Can you work these out from the model? Positions are in its coordinate system, mm. Face numbers are marked on the shaded views. Round coordinates to 2 decimals unless told otherwise and drop trailing zeros. Order: outer loops, then holes, each group sorted by start corner. A loop starts at its lowest first (then second) coordinate and runs counter-clockwise, first axis right, second up. Notation, with made-up numbers: (28.5, 6.25) -> (42.5, 6.25) arc R36 ccw to (42.5, 42.25) -> close; hole circle Ø2 at (11.25, 25.25). An arc over 180 degrees is marked (long way). Use a Markdown table: item, result. Add a question column.
Q1. I'm going to push flat-ended pins straight in: pin 1 Ø8 at (y, z) = (6, -11.5) entering from +X; pin 2 Ø12 at (y, z) = (6, -18) entering from +X; pin 3 Ø3 at (x, y) = (-14, 5.5) entering from -Z. Where does each tip first touch, or does it pass through?
Q2. I need wall thicknesses on line 1 along Z through (x, y) = (0, 15.75); line 2 along X through (y, z) = (9.5, -4); line 3 along Z through (x, y) = (8.5, 17.75). Which ranges of each line are inside material? Lowest first, please. Write a range as [from, to].
Q3. If we section it at C-C on y = 17.5: List the corners of the cut face in (x, z) for me, plus the area to 3 significant figures.
Q4. We'd pull the mould along X, two halves only. Please class the marked faces 1, 2, 3 and 4: +X half, -X half, draft (parallel to the pull), parting line (faces both ways), or undercut.
Q5. If we section it at D-D on x = 38: List the corners of the cut face in (y, z) for me, plus the area to 3 significant figures.
Q6. If we section it at A-A on z = 0: List the corners of the cut face in (x, y) for me, plus the area to 3 significant figures.
Q7. If we section it at B-B on x = 0: List the corners of the cut face in (y, z) for me, plus the area to 3 significant figures.
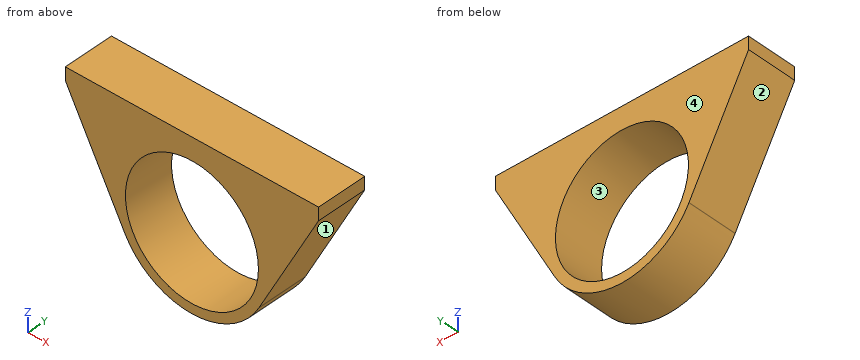
```python
from build123d import *

# Parameters (mm, degrees)
SKETCH1_R           = 30
BOSS_EXTRUDE1_DEPTH = 20
SKETCH2_R           = 26.25
CUT_EXTRUDE1_DEPTH  = 20


with BuildPart() as part:
    # Sketch1 → Boss-Extrude1 (new body)
    with BuildSketch(Plane(origin=(0, 0, 0), x_dir=(1, 0, 0), z_dir=(0, 1, 0))):
        Circle(SKETCH1_R)
        with BuildLine():
            Line((-26.470588235, 14.117647059), (-50, -30))
            Line((-50, -30), (-50, -35))
            Line((-50, -35), (50, -35))
            Line((50, -35), (50, -30))
            Line((50, -30), (26.470588235, 14.117647059))
            ThreePointArc((26.470588235, 14.117647059), (29.104275004, 7.276068751), (30, 0))
            ThreePointArc((30, 0), (-7.276068751, -29.104275004), (-26.470588235, 14.117647059))
        make_face()
    extrude(amount=BOSS_EXTRUDE1_DEPTH)

    # Sketch2 → Cut-Extrude1 (cut)
    with BuildSketch(Plane(origin=(0, 0, 0), x_dir=(1, 0, 0), z_dir=(0, 1, 0))):
        Circle(SKETCH2_R)
    extrude(amount=CUT_EXTRUDE1_DEPTH, mode=Mode.SUBTRACT)


solid = part.part
```
Answer below:
| question | item | result |
|---|---|---|
| 1 | pin 1 | x = 30 |
| 1 | pin 2 | x = 27.6 |
| 1 | pin 3 | z = -27.27 |
| 2 | line 1 | [-30, -26.25], [26.25, 35] |
| 2 | line 2 | [-31.87, -25.94], [25.94, 31.87] |
| 2 | line 3 | [-28.77, -24.84], [24.84, 35] |
| 3 | outline | (-50, 30) -> (-26.47, -14.12) arc R30 ccw to (26.47, -14.12) -> (50, 30) -> (50, 35) -> (-50, 35) -> close; hole circle Ø52.5 at (0, 0) |
| 3 | area | 2,310 mm² |
| 4 | face 1 | +X half |
| 4 | face 2 | -X half |
| 4 | face 3 | undercut |
| 4 | face 4 | draft |
| 5 | outline | (0, 7.5) -> (20, 7.5) -> (20, 35) -> (0, 35) -> close |
| 5 | area | 550 mm² |
| 6 | outline | (-34, 0) -> (-26.25, 0) -> (-26.25, 20) -> (-34, 20) -> close; (26.25, 0) -> (34, 0) -> (34, 20) -> (26.25, 20) -> close |
| 6 | area | 310 mm² |
| 7 | outline | (0, -30) -> (20, -30) -> (20, -26.25) -> (0, -26.25) -> close; (0, 26.25) -> (20, 26.25) -> (20, 35) -> (0, 35) -> close |
| 7 | area | 250 mm² |
